Part model, mm, in its own coordinate system. Face numbers are marked on the shaded views. A direction names the side the tool comes from. Round coordinates to 2 decimals unless told otherwise and drop trailing zeros. Loops run counter-clockwise (first coordinate to the right, second up) from the corner with the lowest first, then second, coordinate; pieces in that order, holes last. Notation, with made-up numbers: (86, 4) - (105, 4) arc R26 cw to (105, 20) - close; hole circle Ø7 at (60.5, -5). An arc over 180 degrees is marked (long way). Put each result on its own line as item: value.
Autodesk Inventor part; units mm, degrees
ref_plane "WorkPlane1" through (0, 0, 0) normal (0, 0, 1) x (1, 0, 0)
ref_plane "MSC_PF1" through (0, 0, 0) normal (1, 0, 0) x (0, 1, 0)
ref_plane "MSC_PT1" through (0, 0, 0) normal (0, 0, -1) x (-1, 0, 0)
ref_plane "WorkPlane1" through (0, 0, 0) normal (0, 0, 1) x (1, 0, 0)
sketch "Sketch1" plane through (0, 0, 0) normal (0, 0, 1) x (1, 0, 0)
  point P0 (0, 0)
sketch "Sketch2" plane through (0, 0, 0) normal (0, 0, 1) x (1, 0, 0)
  line L0 (-6.5, 3.7529) -> (-6.5, -3.7529)
  line L1 (0, 7.5054) -> (-6.5, 3.7529)
  line L2 (6.5, 3.7529) -> (0, 7.5054)
  line L3 (6.5, -3.7529) -> (6.5, 3.7529)
  line L4 (0, -7.5054) -> (6.5, -3.7529)
  line L5 (-6.5, -3.7529) -> (0, -7.5054)
  circle A0 centre (0, 0) radius 6.5 construction
  dimension "d1" = 13
  dimension "d29" = 0
  dimension "d30" = 0
extrude "Extrusion1" add sketch "Sketch2" along normal blind 5.3
sketch "Sketch3" plane through (0, 0, 0) normal (1, 0, 0) x (0, 1, 0)
  line L0 (6.5, 5.3) -> (7.6054, 5.3)
  line L1 (7.6054, 4.6618) -> (6.5, 5.3)
  line L2 (7.6054, 5.3) -> (7.6054, 4.6618)
  line L3 (0, -1.06) -> (0, 6.36)
  line L4 (7.5054, 0) -> (7.5054, 5.3)
  dimension "d25" = 0.1
  dimension "d26" = 0
  dimension "d27" = 60
  dimension "d28" = 6.5
revolve "Revolution1" cut sketch "Sketch3" angle 360 about axis through (0, 0, -10) along (0, 0, 1)
sketch "Sketch4" plane through (0, 0, 0) normal (1, 0, 0) x (0, 1, 0)
  line L0 (0, -20) -> (0, 0)
  line L1 (-4, -20) -> (0, -20)
  line L2 (-4, 0) -> (-4, -20)
  line L3 (0, 0) -> (-4, 0)
  line L4 (0, -20) -> (0, 0)
  line L5 (-4.8, 0) -> (0.8, 0)
  line L6 (0, -24) -> (0, 4)
  dimension "d18" = 4
  dimension "d20" = 20
  dimension "d33" = 0
  dimension "d34" = 0
revolve "Revolution2" add sketch "Sketch4" angle 360 about axis through (0, 0, -20) along (0, 0, -1)
chamfer "Chamfer1" distance 0.625 angle 45 1 edges at (0, 4, -20)
fillet "Fillet1" radius 0.4 1 edges at (0, 4, 0)
thread "Thread1"
ref_plane "MSC_PF1" through (0, 0, 0) normal (1, 0, 0) x (0, 1, 0)
ref_plane "MSC_PT1" through (0, 0, 0) normal (0, 0, -1) x (-1, 0, 0)
equation "\"d22\" = 0.5 * PTC"
equation "\"d23\" = 0.5 * PTC"
equation "\"d24\" = r"
equation "\"d1\" = ParS"
equation "\"d6\" = ParK"
equation "\"b\" = NLG - 2 * PTC"
equation "\"d28\" = 0.5 * ParS"
equation "\"d18\" = 0.5 * NND"
equation "\"d20\" = NLG"
equation "\"NND\" = 8"
equation "\"NLG\" = 20"
equation "\"PTC\" = 1.25"
equation "\"ParK\" = 5.3"
equation "\"ParS\" = 13"
equation "\"msp_es\" = 0.577367 * ParS"
equation "\"r\" = 0.4"
equation "\"THREADDIA\" = NND"
properties part number "ISO 4018 - M8 x 20" material "Steel"
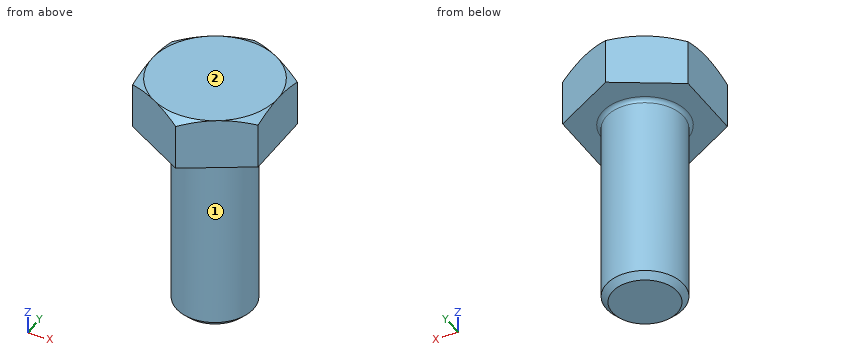
1. Band-saw the part on B-B (z = -6.5). List the corners of the cut face in (x, y).
A:
outline: circle Ø8 at (0, 0)
2. Pin check, flat tips, straight feed: P1, Ø8, axis at y = 5.5, z = -6, coming from the +X side; P2, Ø4, axis at x = 5, y = -4.5, coming from the -Z side; P3, Ø5, axis at x = -2.5, z = -6.5, coming from the +Y side. Stop position of each tip, or through.
A:
P1: stops at x = 3.71
P2: stops at z = 0
P3: stops at y = 4
3. Tool access for the marked faces 1 and 2: list every direction of +Z, -Z, +X, -X, +Y, -Y with a clear straight run to the whole face (end or side of a thin tool).
A:
face 1: -Z
face 2: +Z, +X, -X, +Y, -Y
4. Band-saw the part on A-A (z = 1.5). List the corners of the cut face in (x, y), plus the area to 3 significant figures.
A:
outline: (-6.5, -3.75) - (0, -7.51) - (6.5, -3.75) - (6.5, 3.75) - (0, 7.51) - (-6.5, 3.75) - close
area: 146 mm²
5. Probe line 1 along Z through (x, y) = (-3.5, 3); line 2 along X through (y, z) = (0, -3.25); line 3 along Y through (x, z) = (-1.75, -3.5). List the from-to ranges inside material, lowest first. Write a range as [from, to].
A:
line 1: z = [0, 5.3]
line 2: x = [-4, 4]
line 3: y = [-3.6, 3.6]
